Part print with two shaded views. Sizes in mm from the minimum x, y, z corner. Give positions to 0.01 mm unless a question says otherwise; leave off trailing zeros. Write each loop counter-clockwise with the first axis right and the second up, starting at its lowest first coordinate (ties: lowest second). Pieces come first, ordered by that corner, then holes. Notation, with made-up numbers: (1, 64) - (11, 64) arc R32 ccw to (11, 96) - close; hole circle Ø9 at (-10, -2). An arc over 180 degrees is marked (long way). One line per item, written item: value. Start each with the question number.
(1) Mould opens along X. For the marked faces 1, 2 and 3 say: pulls with the +X half, pulls with the -X half, needs draft (parallel to the pull), parting line crosses it, or undercut.
(2) Probe L1, parallel to Y at x = 6.35, z = 14; L2, parallel to Y at x = 7, z = 15.25; L3, parallel to X at y = 7.5, z = 17.5 (1 decimal). List the from-to ranges inside material, lowest first.
(3) Drop flat-ended pins along their axis: P1, Ø1.5, axis at x = 3, z = 12.5, coming from the -Y side; P2, Ø6, axis at x = 8.5, y = 1.5, coming from the -Z side; P3, Ø1.5, axis at x = 10.5, z = 8, coming from the -Y side. Give the stop position or say it passes through.
(4) Cut at C-C, the plane z = 6.75. List the corners of the cut face in (x, y), and give its area (3 significant figures).
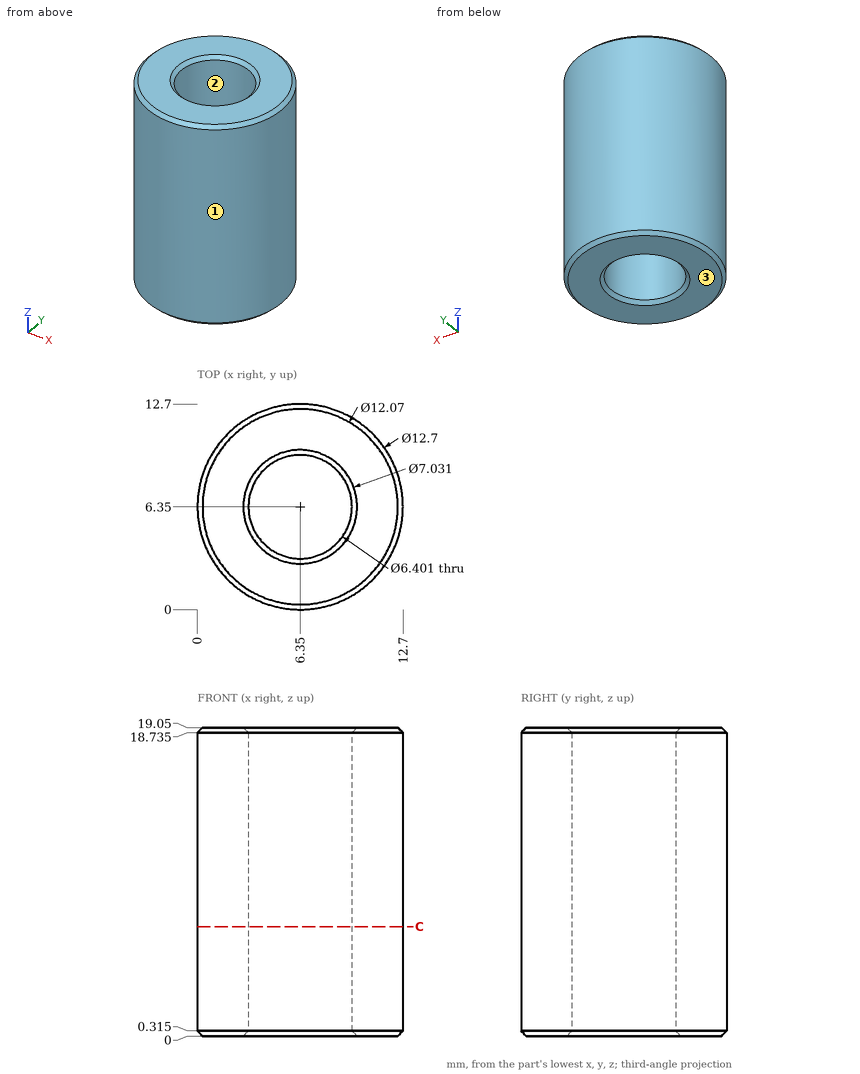
Answers follow:
1. face 1: parting line crosses it
1. face 2: undercut
1. face 3: needs draft
2. L1: y = 0 to 3.15, 9.55 to 12.7
2. L2: y = 0.03 to 3.22, 9.48 to 12.67
2. L3: x = 0.1 to 3.4, 9.3 to 12.6
3. P1: stops at y = 0.56
3. P2: stops at z = 0
3. P3: stops at y = 0.99
4. outline: circle Ø12.7 at (6.35, 6.35); hole circle Ø6.4 at (6.35, 6.35)
4. area: 94.5 mm²
